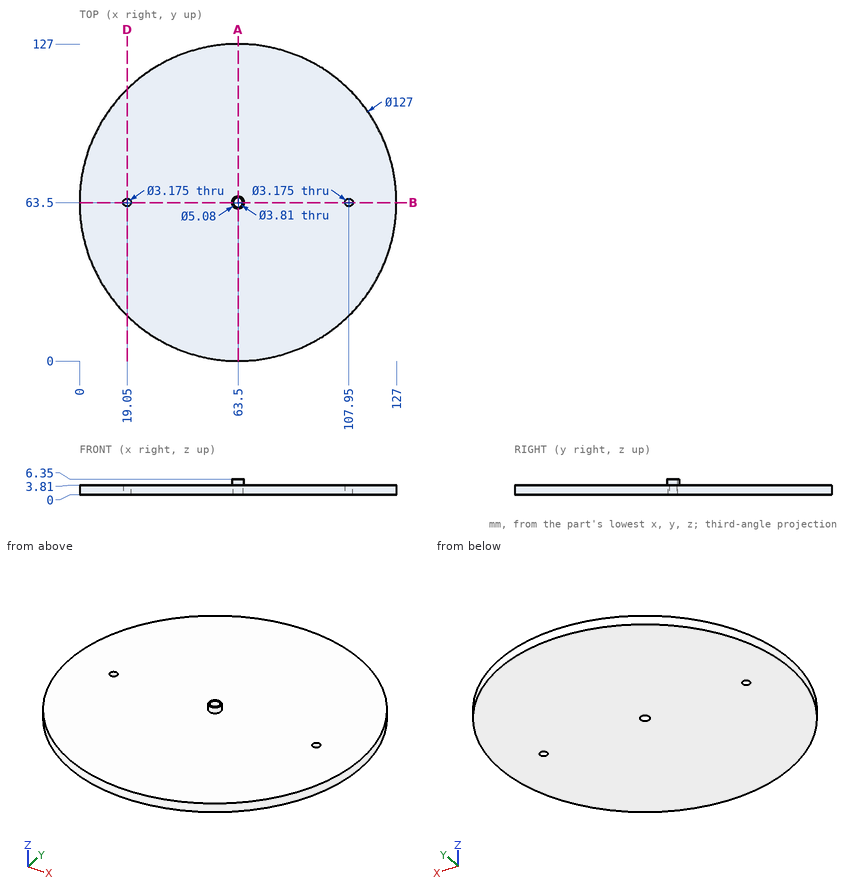
Part print with two shaded views. Sizes in mm from the minimum x, y, z corner. Coordinates: 2 decimals unless noted, no trailing zeros. Write each loop counter-clockwise with the first axis right and the second up, starting at its lowest first coordinate (ties: lowest second). Pieces come first, ordered by that corner, then holes.
1. Band-saw the part on A-A, the plane x = 63.5. Give the cut face in (y, z) (3 decimals).
Answer block:
outline: (0, 0) - (61.595, 0) - (61.595, 6.35) - (60.96, 6.35) - (60.96, 3.81) - (0, 3.81) - close; (65.405, 0) - (127, 0) - (127, 3.81) - (66.04, 3.81) - (66.04, 6.35) - (65.405, 6.35) - close
2. Drill centre lines: probe 1 along Y at (x, z) = (63.5, 4.75) (3 decimals); probe 2 along Z at (x, y) = (57.5, 76); probe 3 along Y at (x, z) = (63.5, 3) (3 decimals). Where is each one in solid material? Low to high.
Answer block:
probe 1: y = 60.96 to 61.595, 65.405 to 66.04
probe 2: z = 0 to 3.81
probe 3: y = 0 to 61.595, 65.405 to 127
3. Band-saw the part on B-B, the plane y = 63.5. Give the number of separate pieces and of enclosed holes in the cut face, and give its area (3 significant figures).
Answer block:
separate pieces: 4
enclosed holes: 0
area: 448 mm2
4. Band-saw the part on D-D, the plane x = 19.05. Give the cut face in (y, z), and give its area (3 significant figures).
Answer block:
outline: (18.15, 0) - (61.91, 0) - (61.91, 3.81) - (18.15, 3.81) - close; (65.09, 0) - (108.85, 0) - (108.85, 3.81) - (65.09, 3.81) - close
area: 333 mm2
5. Drop flat-ended pins along their axis: pin 1 (8 mm diameter, centred on x = 30.5, y = 86.5, fed in from +Z); pin 2 (1 mm diameter, centred on x = 112, y = 41, fed in from -Z); pin 3 (1.5 mm diameter, centred on x = 45, z = 1.5, fed in from +Y). Give the stop position or say it passes through.
Answer block:
pin 1: stops at z = 3.81
pin 2: stops at z = 0
pin 3: stops at y = 124.47
